Geometry check sheet. Reference: the model listing, model coordinates, mm. Give positions to 0.01 mm unless a question says otherwise; leave off trailing zeros. Loops run counter-clockwise (first coordinate to the right, second up) from the corner with the lowest first, then second, coordinate; pieces in that order, holes last. Notation, with made-up numbers: (25.25, 11) - (61.25, 11) arc R11 cw to (61.25, 22) - close; hole circle Ø6 at (27, -11). An arc over 180 degrees is marked (long way). Write item = value, one per line. Start each with the question number.
from build123d import *

# Parameters (mm, degrees)
BOSS_EXTRUDE1_DEPTH = 15
CUT_EXTRUDE1_REACH  = 34.094
SKETCH2_R           = 5


with BuildPart() as part:
    # Sketch1 → Boss-Extrude1 (new body)
    with BuildSketch(Plane.XY):
        with BuildLine():
            Line((-25, 0), (-25, -10))
            Line((-25, -10), (25, -10))
            Line((25, -10), (25, 0))
            ThreePointArc((25, 0), (0, 13.416876048), (-25, 0))
        make_face()
    extrude(amount=BOSS_EXTRUDE1_DEPTH)

    # Sketch2 → Cut-Extrude1 (cut, up to next)
    with BuildSketch(Plane(origin=(0, 0, 0), x_dir=(-1, 0, 0), z_dir=(0, 0, -1)), mode=Mode.PRIVATE) as cut_extrude1_sk1:
        with Locations((0, 3.416876048)):
            Circle(SKETCH2_R)
    cut_extrude1_tool1 = extrude(cut_extrude1_sk1.sketch, amount=-CUT_EXTRUDE1_REACH, mode=Mode.PRIVATE) & part.part
    add(cut_extrude1_tool1.solids().sort_by_distance((0, 3.416876, 0))[0], mode=Mode.SUBTRACT)


solid = part.part
1) Cross-section at D-D on x = 20.5. Enter the section's corners in (y, z), and give its area (3 significant figures).
2) Material ranges on line 1 along X through (y, z) = (6.25, 6.5); line 2 along Y through (x, z) = (4, 11); line 3 along Y through (x, z) = (3, 14), recorded low to high.
3) Cross-section at A-A on x = 0. Enter the section's corners in (y, z).
4) Release check for a two-part mould opening along X. For faces 1 (the face through (25, -5, 7)), 2 (the face through (0.414, 13.414, 7.395)), 3 (the face through (-2.307, -1.019, 7.395)), 4 (the face through (-25, -5, 7)) record: pulls with the +X half, pulls with the -X half, needs draft (parallel to the pull), parting line crosses it, or undercut.
5) Gauge pin test, flat end, axial feed: P1, Ø6, axis at y = 5, z = 8, coming from the -X side. Record the tip position at first contact, or that the pin passes through.
6) Cross-section at B-B on y = 0.75. Enter the section's corners in (x, z), and give its area (3 significant figures).
7) Cross-section at C-C on z = 1.5. Enter the section's corners in (x, y), and give its area (3 significant figures).
Checked values:
q1.outline = (-10, 0) - (5.32, 0) - (5.32, 15) - (-10, 15) - close
q1.area = 230 mm²
q2.line_1 = -19.46 to -4.12, 4.12 to 19.46
q2.line_2 = -10 to 0.42, 6.42 to 13.15
q2.line_3 = -10 to -0.58, 7.42 to 13.27
q3.outline = (-10, 0) - (-1.58, 0) - (-1.58, 15) - (-10, 15) - close; (8.42, 0) - (13.42, 0) - (13.42, 15) - (8.42, 15) - close
q4.face_1 = pulls with the +X half
q4.face_2 = parting line crosses it
q4.face_3 = undercut
q4.face_4 = pulls with the -X half
q5.P1 = -23.55
q6.outline = (-24.49, 0) - (-4.23, 0) - (-4.23, 15) - (-24.49, 15) - close; (4.23, 0) - (24.49, 0) - (24.49, 15) - (4.23, 15) - close
q6.area = 608 mm²
q7.outline = (-25, -10) - (25, -10) - (25, 0) arc R30 ccw to (-25, 0) - close; hole circle Ø10 at (0, 3.42)
q7.area = 893 mm²
